The drawing under review shows one solid part. Ordinate dimensions are in mm from its lowest x, y, z. Coordinates: 2 decimals unless noted, no trailing zeros. One line per question, with ' | ' between items. Start each with the question number.
Q1. Draft analysis for pull direction X (two halves, no side actions). For the marked faces 1, 2 and 3, state which applies: pulls with the +X half, pulls with the -X half, needs draft (parallel to the pull), parting line crosses it, or undercut.
Q2. Wall thickness on probe 1 along Y at (x, z) = (8.5, 17.5); probe 2 along Y at (x, z) = (46, 17.5): over which ranges is each line inside the solid? List them lowest first.
Q3. For P1, Ø10.5, axis at x = 83.5, y = 20, coming from the -Z side, flat-tipped, find the tip position at first contact; note if it passes through.
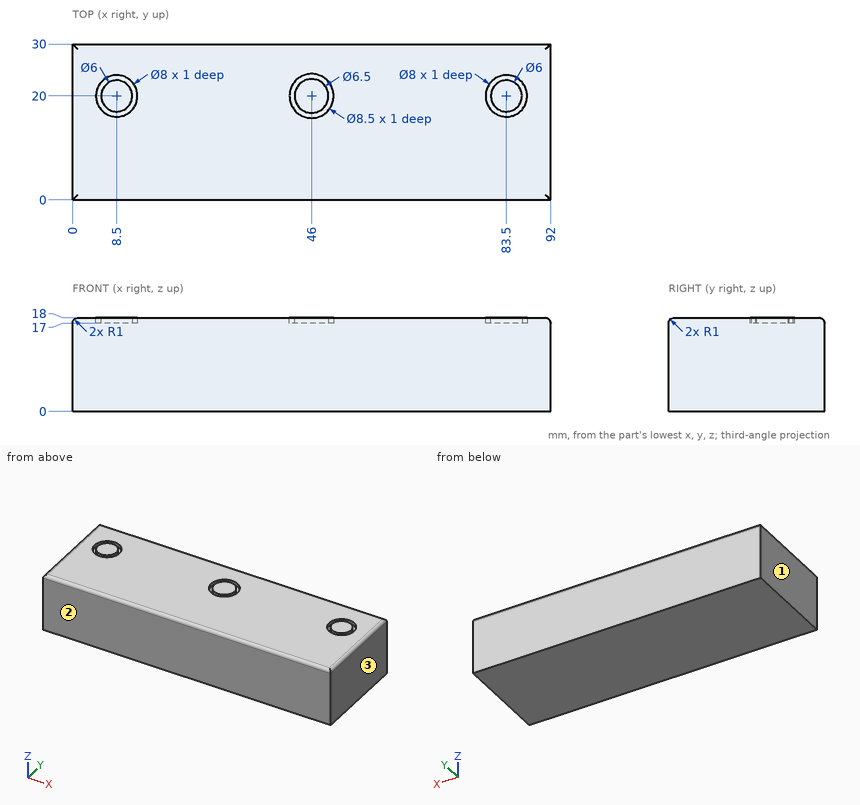
Output values:
1) face 1: pulls with the -X half | face 2: needs draft | face 3: pulls with the +X half
2) probe 1: y = 0.13 to 16, 17 to 23, 24 to 29.87 | probe 2: y = 0.13 to 15.75, 16.75 to 23.25, 24.25 to 29.87
3) P1: stops at z = 0
